```python
from build123d import *

# Parameters (mm, degrees)
BASE_DEPTH          = 3
BASE_DEPTH_BACK     = 6
SKETCH1_R           = 10
SKETCH3_R           = 1.6
HOLE2_DEPTH         = 19.1581212
HOLE2MIRROR_COUNT   = 2
SKETCH4_R           = 1.6
HOLE3_DEPTH         = 19.100993715
SKETCH5_R           = 1.6
CUT_EXTRUDE1_DEPTH  = 19.311666101
SKETCH6_R           = 1.6
CUT_EXTRUDE2_DEPTH  = 19.560472272
SKETCH7_R           = 1.6
CUT_EXTRUDE3_DEPTH  = 19.646604846
FILLET1_R           = 2
EXTRUDE_THIN1_DEPTH = 2


with BuildPart() as part:
    # Sketch1 → base (new, two sides: drawn at the far end of the back side and taken through both)
    with BuildSketch(Plane(origin=(0, 0, 0), x_dir=(1, 0, 0), z_dir=(0, 1, 0)).offset(-BASE_DEPTH_BACK)):
        with Locations(Location((0, 0, 0), (0, 0, 270))):
            Circle(SKETCH1_R)
    extrude(amount=BASE_DEPTH + BASE_DEPTH_BACK)

    # Sketch3 → hole2 (cut, through all)
    with BuildSketch(Plane(origin=(-0.941672921, -1.236067977, 3.685836142), x_dir=(-0.9718935871364875, 0.07382318789513377, -0.22354639834264944), z_dir=(0.23541823021467095, 0.3090169943749464, -0.921459035481267))):
        with Locations(Location((0, 0, 0), (0, 0, 90.062171088))):
            Circle(SKETCH3_R)
    hole2 = extrude(amount=-HOLE2_DEPTH, mode=Mode.SUBTRACT)

    # hole2mirror: hole2 ×2 about axis
    hole2mirror_axis = Axis((0, 5.5, 0), (0, -1, 0))
    for i in range(1, HOLE2MIRROR_COUNT):
        add(hole2.rotate(hole2mirror_axis, i * 360 / HOLE2MIRROR_COUNT), mode=Mode.SUBTRACT)

    # Sketch4 → hole3 (cut, through all)
    with BuildSketch(Plane(origin=(-3.717841, -1.236067977, 0.806098168), x_dir=(-0.19123247894507908, -0.06357892752956036, -0.979483465389136), z_dir=(0.9294602499075393, 0.30901699437494623, -0.20152454200243008))):
        with Locations(Location((0, 0, 0), (0, 0, 90))):
            Circle(SKETCH4_R)
    extrude(amount=-HOLE3_DEPTH, mode=Mode.SUBTRACT)

    # Sketch5 → Cut-Extrude1 (cut, through all)
    with BuildSketch(Plane(origin=(3.671965021, -1.093066116, -1.149730122), x_dir=(0.2754858058396647, -0.08200628219437099, 0.9578008876909271), z_dir=(-0.9179912552075574, 0.27326652891267317, 0.2874325304110031))):
        with Locations(Location((0, 0, 0), (0, 0, 4.890463))):
            Circle(SKETCH5_R)
    extrude(amount=-CUT_EXTRUDE1_DEPTH, mode=Mode.SUBTRACT)

    # Sketch6 → Cut-Extrude2 (cut, through all)
    with BuildSketch(Plane(origin=(2.875583134, -1.236067977, 2.490613899), x_dir=(-0.5720437997755544, 0.24589274231852376, 0.782497699941298), z_dir=(-0.7188957835464718, 0.30901699437494723, -0.6226534747245682))):
        with Locations(Location((0, 0, 0), (0, 0, 345.016140445))):
            Circle(SKETCH6_R)
    extrude(amount=-CUT_EXTRUDE2_DEPTH, mode=Mode.SUBTRACT)

    # Sketch7 → Cut-Extrude3 (cut, through all)
    with BuildSketch(Plane(origin=(-2.670502563, -1.093066116, -2.770130417), x_dir=(0.7444971483747472, -0.2450509606833859, -0.6210265877802813), z_dir=(0.6676256406564008, 0.2732665289126714, 0.6925326043690294))):
        with Locations(Location((0, 0, 0), (0, 0, 14.758597305))):
            Circle(SKETCH7_R)
    extrude(amount=-CUT_EXTRUDE3_DEPTH, mode=Mode.SUBTRACT)

    # Fillet1
    fillet1_edges = [part.edges().sort_by_distance(p)[0] for p in [
        (0, 3, -10),
    ]]
    fillet(fillet1_edges, radius=FILLET1_R)

    # Sketch9 → Extrude-Thin1 (add)
    with BuildSketch(Plane(origin=(0, 3, 0), x_dir=(1, 0, 0), z_dir=(0, 1, 0))):
        Polygon((-4.40005736, 3.518760981), (-0.246688962, -1.237871846), (6.097894842, 1.902273668), (5.210740629, 3.694746095), (0.246688962, 1.237871846), (-2.893541545, 4.834211512), align=None)
    extrude(amount=EXTRUDE_THIN1_DEPTH)


solid = part.part
```
Can you work these out from the model? Positions are in its coordinate system, mm. A direction names the side the tool comes from. Give positions to 0.01 mm unless a question says otherwise; leave off trailing zeros. Loops run counter-clockwise (first coordinate to the right, second up) from the corner with the lowest first, then second, coordinate; pieces in that order, holes last. Notation, with made-up numbers: M 44,-8 L 95,-8 A6 cw 95,-1 Z; hole C 52.5,-18 d8. An arc over 180 degrees is marked long. One line per item, written item: value.
(1) Will these pins go through, and if not, where does the flat tip stop? pin 1 (8 mm diameter, centred on x = 1.5, z = 1.5, fed in from +Y); pin 2 (2 mm diameter, centred on y = -3, z = 5.5, fed in from +X); pin 3 (5 mm diameter, centred on x = -2.5, y = 3, fed in from -Z); pin 4 (5 mm diameter, centred on y = -0.5, z = -4, fed in from +X).
Returned:
pin 1: y = 5
pin 2: x = 8.93
pin 3: z = -9.96
pin 4: x = 9.89
(2) Suppose I cut it at D-D on y = 2.5. List the corners of the cut face in (x, z) for me, plus the area to 3 significant figures.
Returned:
outline: C 0,0 d18.65
area: 273 mm^2
(3) Which directions (+Z, -Z, +X, -X, +Y, -Y) give clear straight access to the entire face, cutting with the end or side of a thin tool? Please do faces 1 (the face through (2.8, 4, -2.5)), 2 (the face through (2.88, 3.99, -0.31)), 3 (the face through (-2.35, 3.99, -1.17)), 4 (the face through (0.92, -1.259, -3.684)).
Returned:
face 1: -Z, +Y
face 2: +Z, +X, +Y
face 3: +Z, -X, +Y
face 4: none
(4) Suppose I cut it at B-B on x = 0. Count the separate pieces of the cut face and the enclosed holes in it, plus the area to 3 significant figures.
Returned:
separate pieces: 1
enclosed holes: 2
area: 174 mm^2
(5) Suppose I cut it at A-A on y = 4.25. List the corners of the cut face in (x, z) for me, plus the area to 3 significant figures.
Returned:
outline: M -4.4,-3.52 L -2.89,-4.83 L 0.25,-1.24 L 5.21,-3.69 L 6.1,-1.9 L -0.25,1.24 Z
area: 23.7 mm^2
(6) We'd pull the mould along Z, two halves only. Please class faces 5 (the face through (2.895, -1.215, 2.478)), 6 (the face through (-0.92, -1.259, 3.684)), 7 (the face through (-1.3, 3.99, -3.01)), 8 (the face through (0, 3, 2)): released by +Z, released by -Z, zero draft, split by the parting line, or undercut.
Returned:
face 5: undercut
face 6: undercut
face 7: released by -Z
face 8: zero draft
(7) I need wall thicknesses on line 1 (Z direction, x = -4.5, y = -1.25); line 2 (Z direction, x = -7.75, y = -3.25); line 3 (Z direction, x = -6.25, y = -2.75). Which ranges of each line are inside material? Lowest first, please.
Returned:
line 1: -8.93 to -6.54, -2.37 to -0.66, 2.58 to 8.93
line 2: -5.85 to 0.23, 3.22 to 6.32
line 3: -4.35 to -0.1, 2.9 to 7.81
